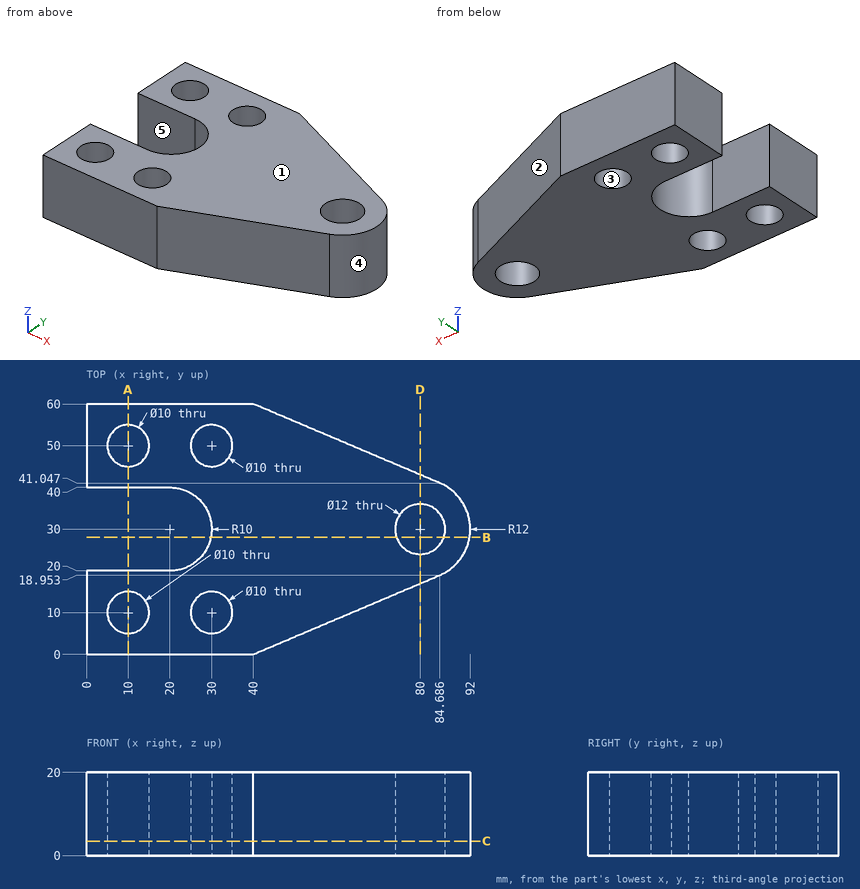
Here's the drawing with two shaded views (mm, measured from the low corner). I have some questions. A direction names the side the tool comes from. Coordinates: 2 decimals unless noted, no trailing zeros. Loops run counter-clockwise (first coordinate to the right, second up) from the corner with the lowest first, then second, coordinate; pieces in that order, holes last. Notation, with made-up numbers: M 44,88.5 L 80,88.5 A23 cw 80,122.5 Z; hole C -5,84.5 d2. An arc over 180 degrees is marked long. Put each result on its own line as item: value. Start each with the question number.
(1) Which directions (+Z, -Z, +X, -X, +Y, -Y) give clear straight access to the entire face, cutting with the end or side of a thin tool? Please do the marked faces 4 and 5.
(2) Imagine slicing it at D-D on x = 80. List the corners of the cut face in (y, z) for me (1 decimal), and give its area (3 significant figures).
(3) I need wall thicknesses on probe 1 along Y at (x, z) = (10, 11); probe 2 along X at (y, z) = (11, 8.75) (1 decimal); probe 3 along Y at (x, z) = (12, 7.25). Which ranges of each line are inside material? Lowest first, please.
(4) We'd pull the mould along Y, two halves only. Please class the marked faces 1, 2 and 3: +Y half, -Y half, draft (parallel to the pull), parting line (faces both ways), or undercut.
(5) Imagine slicing it at A-A on x = 10. List the corners of the cut face in (y, z) for me, and give its area (3 significant figures).
(6) Imagine slicing it at C-C on z = 3.5. List the corners of the cut face in (x, y) for me (1 decimal), and give its area (3 significant figures).
(7) Will these pins go through, and if not, where does the flat tip stop? pin 1 Ø8 at (x, y) = (10, 10) entering from +Z; pin 2 Ø1 at (x, z) = (56.5, 3) entering from -Y; pin 3 Ø8 at (y, z) = (32.5, 5) entering from -X; pin 4 Ø2 at (y, z) = (53, 6) entering from +X (1 decimal).
(8) Imagine slicing it at B-B on y = 28. List the corners of the cut face in (x, z) for me, and give its area (3 significant figures).
Worked answers:
1. face 4: +Z, -Z, +X
1. face 5: +Z, -Z, -X
2. outline: M 17,0 L 24,0 L 24,20 L 17,20 Z; M 36,0 L 43,0 L 43,20 L 36,20 Z
2. area: 281 mm2
3. probe 1: y = 0 to 5, 15 to 20, 40 to 45, 55 to 60
3. probe 2: x = 0 to 5.1, 14.9 to 25.1, 34.9 to 65.9
3. probe 3: y = 0 to 5.42, 14.58 to 20, 40 to 45.42, 54.58 to 60
4. face 1: draft
4. face 2: +Y half
4. face 3: undercut
5. outline: M 0,0 L 5,0 L 5,20 L 0,20 Z; M 15,0 L 20,0 L 20,20 L 15,20 Z; M 40,0 L 45,0 L 45,20 L 40,20 Z; M 55,0 L 60,0 L 60,20 L 55,20 Z
5. area: 400 mm2
6. outline: M 0,0 L 40,0 L 84.7,19 A12 ccw 84.7,41 L 40,60 L 0,60 L 0,40 L 20,40 A10 cw 20,20 L 0,20 Z; hole C 10,10 d10; hole C 10,50 d10; hole C 30,10 d10; hole C 30,50 d10; hole C 80,30 d12
6. area: 3,370 mm2
7. pin 1: passes through
7. pin 2: stops at y = 6.79
7. pin 3: stops at x = 27.6
7. pin 4: stops at x = 58.9
8. outline: M 29.8,0 L 74.34,0 L 74.34,20 L 29.8,20 Z; M 85.66,0 L 91.83,0 L 91.83,20 L 85.66,20 Z
8. area: 1,010 mm2
